For this review, take the finished solid that the model builds, in its own axes (mm). A direction names the side the tool comes from. Coordinates: 2 decimals unless noted, no trailing zeros. Loops run counter-clockwise (first coordinate to the right, second up) from the corner with the lowest first, then second, coordinate; pieces in that order, holes last. Notation, with made-up numbers: (63.5, 49) - (118.5, 49) arc R17 ccw to (118.5, 71) - close; hole circle Ø8 at (61, 42). An arc over 180 degrees is marked (long way). Answer as a JSON object with one key per item and string values. Group by question number.
Item 1: Clearance check with flat-ended pins moving along their axes: pin 1 (1 mm diameter, centred on y = -46.5, z = 6.5, fed in from -X); pin 2 (1.5 mm diameter, centred on y = -22.5, z = 14.5, fed in from +X); pin 3 (1.5 mm diameter, centred on y = -30, z = 7, fed in from +X). State where each tip first meets the part, or that it passes through.
Item 2: Mouldability with a two-part tool opening along X and no side actions: class faces 1 (the cylindrical face through (9.47, -54.52, 9.39)), 2 (the flat face through (120, -32, 9.525)), 3 (the flat face through (489, -63.5, 9)) as released by +X, released by -X, zero draft, split by the parting line, or undercut.
Item 3: To check wall thickness, follow line 1 (Y direction, x = 723.9, z = 6.75); line 2 (Z direction, x = 609.5, y = -41) (3 decimals); line 3 (Y direction, x = 229, z = 2.5). State the ranges of each line that lie inside material, in increasing order.
Item 4: Tool access review of faces 4 (the flat face through (482, -32, 9.525)), 5 (the flat face through (489, -31, 19.05)): name each direction out of +Z, -Z, +X, -X, +Y, -Y from which nothing blocks a thin tool from reaching the whole face with its end or side.
Item 5: We need section A-A (x = 482.6). Give the boundary of the cut face in (y, z) (3 decimals).
Item 6: We need section B-B (z = 5.75). Give the boundary of the cut face in (x, y).
from build123d import *

# Parameters (mm, degrees)
BOSS_EXTRUDE1_DEPTH = 19.05
SKETCH3_R           = 16.66875
CUT_EXTRUDE1_DEPTH  = 9.525


with BuildPart() as part:
    # Sketch2 → Boss-Extrude1 (new body)
    with BuildSketch(Plane.XY):
        with BuildLine():
            Line((31.496, 0), (933.704, 0))
            ThreePointArc((933.704, 0), (955.97503518, -9.22496482), (965.2, -31.496))
            Line((965.2, -31.496), (965.2, -32.004))
            ThreePointArc((965.2, -32.004), (955.97503518, -54.27503518), (933.704, -63.5))
            Line((933.704, -63.5), (31.496, -63.5))
            ThreePointArc((31.496, -63.5), (9.22496482, -54.27503518), (0, -32.004))
            Line((0, -32.004), (0, -31.496))
            ThreePointArc((0, -31.496), (9.22496482, -9.22496482), (31.496, 0))
        make_face()
    extrude(amount=BOSS_EXTRUDE1_DEPTH)

    # Sketch3 → Cut-Extrude1 (cut)
    with BuildSketch(Plane.XY):
        with Locations((844.55, -31.75)):
            Circle(SKETCH3_R)
        with Locations((723.9, -31.75)):
            Circle(SKETCH3_R)
        with Locations((603.25, -31.75)):
            Circle(SKETCH3_R)
        with Locations((482.6, -31.75)):
            Circle(SKETCH3_R)
        with Locations((361.95, -31.75)):
            Circle(SKETCH3_R)
        with Locations((241.3, -31.75)):
            Circle(SKETCH3_R)
        with Locations((120.65, -31.75)):
            Circle(SKETCH3_R)
    extrude(amount=CUT_EXTRUDE1_DEPTH, mode=Mode.SUBTRACT)


solid = part.part
Check sheet entries:
{
 "1": {"pin 1": "stops at x = 3.28", "pin 2": "stops at x = 964.1", "pin 3": "stops at x = 965.19"},
 "2": {"face 1": "released by -X", "face 2": "undercut", "face 3": "zero draft"},
 "3": {"line 1": "y = -63.5 to -48.42, -15.08 to 0", "line 2": "z = 9.525 to 19.05", "line 3": "y = -63.5 to -43, -20.5 to 0"},
 "4": {"face 4": "-Z", "face 5": "+Z, +X, -X, +Y, -Y"},
 "5": {"outline": "(-63.5, 0) - (-48.419, 0) - (-48.419, 9.525) - (-15.081, 9.525) - (-15.081, 0) - (0, 0) - (0, 19.05) - (-63.5, 19.05) - close"},
 "6": {"outline": "(0, -32) arc R31.5 ccw to (31.5, -63.5) - (933.7, -63.5) arc R31.5 ccw to (965.2, -32) - (965.2, -31.5) arc R31.5 ccw to (933.7, 0) - (31.5, 0) arc R31.5 ccw to (0, -31.5) - close; hole circle Ø33.34 at (120.65, -31.75); hole circle Ø33.34 at (241.3, -31.75); hole circle Ø33.34 at (361.95, -31.75); hole circle Ø33.34 at (482.6, -31.75); hole circle Ø33.34 at (603.25, -31.75); hole circle Ø33.34 at (723.9, -31.75); hole circle Ø33.34 at (844.55, -31.75)"}
}
